from build123d import *

# Parameters (mm, degrees)
SKETCH1_W               = 25
SKETCH1_H               = 16
BOSS_EXTRUDE1_DEPTH     = 20
SKETCH6_R               = 17.5
BOSS_EXTRUDE4_DEPTH     = 65
CUT_EXTRUDE1_DEPTH      = 65
CUT_EXTRUDE1_DEPTH_BACK = 40
SKETCH2_W               = 14
SKETCH2_H               = 15
SKETCH3_R               = 1
CUT_EXTRUDE2_DEPTH      = 10
SKETCH7_R               = 15.5
CUT_EXTRUDE3_DEPTH      = 30


with BuildPart() as part:
    # Sketch1 → Boss-Extrude1 (new body)
    with BuildSketch(Plane(origin=(0, 0, 0), x_dir=(1, 0, 0), z_dir=(0, 1, 0))):
        with Locations((3.281818182, -1.972727273)):
            Rectangle(SKETCH1_W, SKETCH1_H)
    extrude(amount=BOSS_EXTRUDE1_DEPTH)

    # Sketch6 → Boss-Extrude4 (add)
    with BuildSketch(Plane(origin=(0, 0, 0), x_dir=(1, 0, 0), z_dir=(0, 1, 0))):
        with Locations(Location((3.872523773, -1.953116283, 0), (0, 0, 270))):
            Circle(SKETCH6_R)
    extrude(amount=BOSS_EXTRUDE4_DEPTH)

    # Sketch2 → Cut-Extrude1 (cut, two sides: drawn at the far end of the back side and taken through both)
    with BuildSketch(Plane.ZY.offset(9.218181818).offset(-CUT_EXTRUDE1_DEPTH_BACK)):
        with Locations((1.972727273, 11.5)):
            Rectangle(SKETCH2_W, SKETCH2_H)
    extrude(amount=CUT_EXTRUDE1_DEPTH + CUT_EXTRUDE1_DEPTH_BACK, mode=Mode.SUBTRACT)

    # Sketch3 → Cut-Extrude2 (cut)
    with BuildSketch(Plane(origin=(0, 0, 0), x_dir=(-1, 0, 0), z_dir=(0, -1, 0))):
        with Locations(Location((-9.781818182, -1.972727273, 0), (0, 0, 90))):
            Circle(SKETCH3_R)
        with Locations(Location((0.218181818, -1.972727273, 0), (0, 0, 90))):
            Circle(SKETCH3_R)
    extrude(amount=-CUT_EXTRUDE2_DEPTH, mode=Mode.SUBTRACT)

    # Sketch7 → Cut-Extrude3 (cut)
    with BuildSketch(Plane(origin=(0, 65, 0), x_dir=(1, 0, 0), z_dir=(0, 1, 0))):
        with Locations(Location((3.872523773, -1.953116283, 0), (0, 0, 270))):
            Circle(SKETCH7_R)
    extrude(amount=-CUT_EXTRUDE3_DEPTH, mode=Mode.SUBTRACT)


solid = part.part
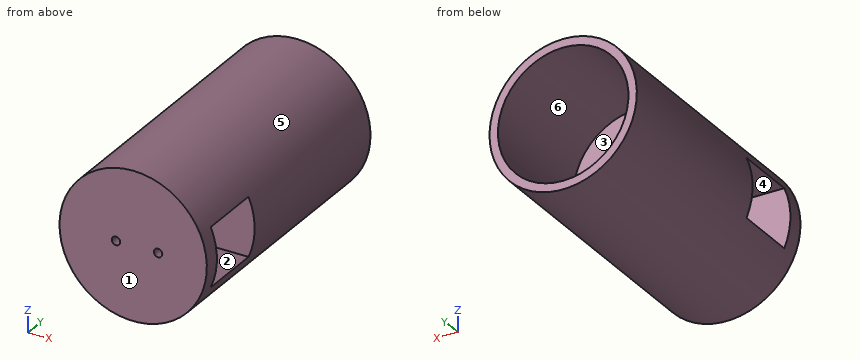
Can you work these out from the model? Positions are in its coordinate system, mm. Face numbers are marked on the shaded views. A direction names the side the tool comes from. Coordinates: 2 decimals unless noted, no trailing zeros. Order: outer loops, then holes, each group sorted by start corner. A loop starts at its lowest first (then second) coordinate and runs counter-clockwise, first axis right, second up. Notation, with made-up numbers: (55.5, -9.75) - (68.5, -9.75) arc R20 ccw to (68.5, 2.25) - close; hole circle Ø7 at (36.5, 80.25). An arc over 180 degrees is marked (long way). Answer as a JSON object with one key per item and string values. Group by question number.
Q1. On a 3-axis mill with a long thin cutter (end or side, diameter ignored), from which of +Z, -Z, +X, -X, +Y, -Y can I reach the whole of each face in a straight line? I mean the marked faces 4, 5 and 6. Say none if no direction works.
Q2. Imagine slicing it at D-D (z = 12.5). Please give me the cut outline in (x, y).
Q3. Imagine slicing it at B-B (x = 18.5). Please give me the cut outline in (y, z), and give its area (3 significant figures).
Q4. I need wall thicknesses on line 1 (Y direction, x = 1, z = -2); line 2 (Z direction, x = 4, y = 11.5); line 3 (Z direction, x = 3.5, y = 32). Which ranges of each line are inside material? Lowest first, please. Write a range as from..to.
Q5. Will these pins go through, and if not, where does the flat tip stop? P1, Ø4, axis at x = 5, z = 2.5, coming from the +Y side; P2, Ø4, axis at x = -5, y = 45.5, coming from the +Z side; P3, Ø3, axis at y = 33, z = 0, coming from the +X side.
Q6. Imagine slicing it at A-A (z = -4). Please give me the cut outline in (x, y), and give its area (3 significant figures).
Q7. We'd pull the mould along Y, two halves only. Please class the marked faces 1, 2 and 3: +Y half, -Y half, draft (parallel to the pull), parting line (faces both ways), or undercut.
Q8. Imagine slicing it at C-C (y = 9). Please give me the cut outline in (x, z), and give its area (3 significant figures).
Determined:
{
 "1": {"face 4": "+X, -X", "face 5": "+Y, -Y", "face 6": "+Y"},
 "2": {"outline": "(-10.09, 0) - (17.84, 0) - (17.84, 65) - (15.23, 65) - (15.23, 35) - (-7.49, 35) - (-7.49, 65) - (-10.09, 65) - close"},
 "3": {"outline": "(0, -7.65) - (65, -7.65) - (65, -3.17) - (35, -3.17) - (35, 7.08) - (65, 7.08) - (65, 11.56) - (0, 11.56) - close; hole (4, -5.03) - (19, -5.03) - (19, 8.97) - (4, 8.97) - close", "area": "731 mm2"},
 "4": {"line 1": "y = 0..4, 19..35", "line 2": "z = -15.55..-5.03, 8.97..19.45", "line 3": "z = -15.54..19.45"},
 "5": {"P1": "stops at y = 35", "P2": "stops at z = 18.05", "P3": "stops at x = 21.37"},
 "6": {"outline": "(-12.58, 0) - (20.33, 0) - (20.33, 4) - (-12.58, 4) - close; (-12.58, 19) - (20.33, 19) - (20.33, 65) - (18.18, 65) - (18.18, 35) - (-10.44, 35) - (-10.44, 65) - (-12.58, 65) - close", "area": "787 mm2"},
 "7": {"face 1": "-Y half", "face 2": "undercut", "face 3": "+Y half"},
 "8": {"outline": "(-12.18, -5.03) arc R17.5 ccw to (19.92, -5.03) - close; (-12.16, 8.97) - (19.9, 8.97) arc R17.5 ccw to start", "area": "486 mm2"}
}
